CAD build for the part. Positions are in the model's coordinates, mm. A direction names the side the tool comes from. Coordinates: 2 decimals unless noted, no trailing zeros. Loops run counter-clockwise (first coordinate to the right, second up) from the corner with the lowest first, then second, coordinate; pieces in that order, holes last.
1) Which spindle directions (+Z, -Z, +X, -X, +Y, -Y) get a long thin tool onto all of the face, cutting with end or side? Do faces 1 (the flat face through (-20.891, -176, 4)), 2 (the flat face through (-38, -115.79, 4)), 3 (the flat face through (-24.701, -35, 4)). Say none if no direction does.
2) Wall check: line 1 along Y through (x, z) = (-29, 6); line 2 along X through (y, z) = (-92.5, 6.5); line 3 along X through (y, z) = (-120, 2.5). Give the ranges that are in metal, low to high.
3) Pin check, flat tips, straight feed: pin 1 Ø2.5 at (x, z) = (-40.5, 2.5) entering from -Y; pin 2 Ø1.1 at (x, z) = (-19, 2.5) entering from -Y; pin 3 Ø4 at (y, z) = (-164.5, 3) entering from -X. Stop position of each tip, or through.
4) Saw through at B-B, the plane x = -44.5. Write the cut outline in (y, z).
5) Saw through at A-A, the plane z = 4.5. Write the cut outline in (x, y), and give its area (3 significant figures).
6) Saw through at C-C, the plane y = -10. Write the cut outline in (x, z).
```python
from build123d import *

# Parameters (mm, degrees)
F0_W     = 26.502896
F0_H     = 148.872193
F1_DEPTH = 7.62
F2_W     = 13.007119
F2_H     = 7.62
F3_DEPTH = 7.62
F4_W     = 3.81
F4_H     = 7.62
F5_DEPTH = 127


with BuildPart() as f1:
    # F0 (on Top) → F1 (new body)
    with BuildSketch(Plane.XY):
        with Locations((-37.95266, -41.353592)):
            Rectangle(F0_W, F0_H)
    extrude(amount=F1_DEPTH)

    # F2 (on face) → F3 (join)
    with BuildSketch(Plane.YZ.offset(-24.701212)):
        with Locations((-106.736221, 3.81)):
            Rectangle(F2_W, F2_H)
    extrude(amount=F3_DEPTH)

    # F4 (on face) → F5 (join)
    with BuildSketch(Plane.XZ.offset(113.23978)):
        with Locations((-22.796212, 3.81)):
            Rectangle(F4_W, F4_H)
    extrude(amount=F5_DEPTH)


solid = f1.part
```
Data:
1. face 1: +Z, -Z, +X, -Y
1. face 2: +Z, -Z, -X, -Y
1. face 3: +Z, -Z, +X, +Y
2. line 1: y = -115.79 to 33.08
2. line 2: x = -51.2 to -24.7
2. line 3: x = -24.7 to -20.89
3. pin 1: stops at y = -115.79
3. pin 2: stops at y = -113.24
3. pin 3: stops at x = -24.7
4. outline: (-115.79, 0) - (33.08, 0) - (33.08, 7.62) - (-115.79, 7.62) - close
5. outline: (-51.2, -115.79) - (-24.7, -115.79) - (-24.7, -240.24) - (-20.89, -240.24) - (-20.89, -113.24) - (-17.08, -113.24) - (-17.08, -100.23) - (-24.7, -100.23) - (-24.7, 33.08) - (-51.2, 33.08) - close
5. area: 4,530 mm2
6. outline: (-51.2, 0) - (-24.7, 0) - (-24.7, 7.62) - (-51.2, 7.62) - close
